Autodesk Inventor part; units mm, degrees
ref_plane "YZ Plane" through (0, 0, 0) normal (1, 0, 0) x (0, 1, 0)
ref_plane "XZ Plane" through (0, 0, 0) normal (0, 1, 0) x (-1, 0, 0)
ref_plane "XY Plane" through (0, 0, 0) normal (0, 0, 1) x (1, 0, 0)
sketch "スケッチ1" plane through (0, 0, 0) normal (0, 0, 1) x (1, 0, 0)
  line L0 (-341.5, 417.85) -> (341.5, 417.85)
  line L1 (341.5, 417.85) -> (341.5, -417.85)
  line L2 (341.5, -417.85) -> (-341.5, -417.85)
  line L3 (-341.5, -417.85) -> (-341.5, 417.85)
  line L4 (-478.1, 0) -> (478.1, 0)
  line L5 (0, -584.99) -> (0, 584.99)
  point P0 (0, 0)
  point P1 (341.5, 0)
  point P2 (0, 417.85)
  dimension "d2" = 835.7
  dimension "d3" = 683
extrude "押し出し1" add sketch "スケッチ1" along normal blind 1357
sketch "スケッチ3" plane through (0, 0, 0) normal (0, 0, 1) x (1, 0, 0)
  line L0 (-171.5, 417.85) -> (171.5, 417.85)
  line L1 (171.5, 417.85) -> (341.5, -132.15)
  line L2 (341.5, -132.15) -> (341.5, -166.8)
  line L3 (341.5, -166.8) -> (135, -417.85)
  line L4 (-341.5, 417.85) -> (341.5, 417.85)
  line L5 (341.5, 417.85) -> (341.5, -417.85)
  line L6 (341.5, -417.85) -> (-341.5, -417.85)
  line L7 (0, -595.6665) -> (0, 649.0488)
  line L8 (135, -417.85) -> (0, -417.85)
  line L9 (-341.5, -417.85) -> (341.5, -417.85)
  line L10 (-171.5, 417.85) -> (-341.5, -132.15)
  line L11 (-341.5, -132.15) -> (-341.5, -166.8)
  line L12 (-341.5, -166.8) -> (-135, -417.85)
  line L13 (-135, -417.85) -> (0, -417.85)
  line L14 (341.5, 417.85) -> (-341.5, 417.85)
  line L15 (171.5, 417.85) -> (341.5, 417.85)
  line L16 (341.5, 417.85) -> (341.5, -132.15)
  line L17 (341.5, -417.85) -> (341.5, 417.85)
  line L18 (341.5, -166.8) -> (341.5, -417.85)
  line L19 (341.5, -417.85) -> (135, -417.85)
  line L20 (-135, -417.85) -> (-341.5, -417.85)
  line L21 (-341.5, -417.85) -> (-341.5, -166.8)
  line L22 (-341.5, 417.85) -> (-341.5, -417.85)
  line L23 (-171.5, 417.85) -> (-341.5, 417.85)
  line L24 (-341.5, -132.15) -> (-341.5, 417.85)
  point P0 (0, 0)
  point P1 (0, 417.85)
  dimension "d9" = 343
  dimension "d10" = 34.65
  dimension "d11" = 550
  dimension "d12" = 206.5
extrude "押し出し2" cut sketch "スケッチ3" along normal through all both and the other way through all contours L10 L22 L4 | L4 L5 L1 | L12 L6 L21 | L3 L5 L6
sketch "スケッチ5" plane through (0, 0, 1357) normal (0, 0, 1) x (1, 0, 0)
  line L0 (-171.5, 417.85) -> (-341.5, -132.15)
  line L1 (-341.5, -132.15) -> (-171.5, 417.85)
  line L2 (171.5, 417.85) -> (-171.5, 417.85)
  line L3 (-171.5, 417.85) -> (171.5, 417.85)
  line L4 (341.5, -132.15) -> (171.5, 417.85)
  line L5 (171.5, 417.85) -> (341.5, -132.15)
  line L6 (341.5, -132.15) -> (-341.5, -132.15)
  point P0 (0, 0)
extrude "押し出し3" cut sketch "スケッチ5" against normal blind 1337
sketch "スケッチ6" plane through (-341.5, -132.15, 1357) normal (0, 1, 0) x (1, 0, 0)
  line L0 (0, 1265.7) -> (0, 665.7)
  line L1 (0, 665.7) -> (76.7, 665.7)
  line L2 (76.7, 665.7) -> (0, 1265.7)
  line L3 (0, 1357) -> (170, 1357)
  line L4 (0, 0) -> (0, 1337)
  line L5 (341.5, 1357) -> (341.5, 1610.7019)
  line L6 (683, 1265.7) -> (683, 665.7)
  line L7 (683, 665.7) -> (606.3, 665.7)
  line L8 (606.3, 665.7) -> (683, 1265.7)
  line L9 (0, 665.7) -> (76.7, 665.7)
  line L10 (0, 665.7) -> (0, 0)
  line L11 (0, 1357) -> (0, 0)
  line L12 (76.7, 665.7) -> (122.641, 0)
  line L13 (206.5, 0) -> (206.5, 1357)
  line L14 (0, 0) -> (122.641, 0)
  line L15 (683, 0) -> (0, 0)
  line L16 (683, 665.7) -> (606.3, 665.7)
  line L17 (683, 665.7) -> (606.3, 665.7)
  line L18 (683, 665.7) -> (683, 0)
  line L19 (606.3, 665.7) -> (560.359, 0)
  line L20 (683, 0) -> (560.359, 0)
  point P0 (683, 0)
  dimension "d17" = 91.3
  dimension "d18" = 600
  dimension "d19" = 76.7
  dimension "d21" = 45.941
extrude "押し出し4" cut sketch "スケッチ6" against normal through all
sketch "スケッチ7" plane through (0, 0, 0) normal (1, 0, 0) x (0, 1, 0)
  line L0 (-315.8994, 1357) -> (-417.85, 1357)
  line L1 (-371.05, 1357) -> (-417.85, 1357)
  line L2 (-417.85, 1357) -> (-417.85, 799.8485)
  line L3 (-417.85, 1357) -> (-417.85, 0)
  line L4 (-417.85, 799.8485) -> (-371.05, 862.4972)
  line L5 (-371.05, 862.4972) -> (-371.05, 1357)
  line L6 (-315.8994, 1357) -> (-260.0471, 691.3)
  line L7 (-417.85, 0) -> (-417.85, 1357)
  point P0 (0, 0)
  dimension "d25" = 143.239
  dimension "d26" = 46.8
extrude "押し出し5" cut sketch "スケッチ7" along normal through all both and the other way through all
sketch "スケッチ8" plane through (0, 0, 0) normal (1, 0, 0) x (0, 1, 0)
  line L0 (-132.15, 20) -> (417.85, 20)
  line L1 (167.85, 20) -> (-132.15, 252.8315)
  line L2 (-132.15, 91.3) -> (-132.15, 691.3)
  line L3 (-132.15, 20) -> (-132.15, 91.3)
  line L4 (-132.15, 252.8315) -> (-132.15, 20)
  line L5 (-132.15, 20) -> (167.85, 20)
  point P0 (0, 0)
  dimension "d29" = 37.815
  dimension "d30" = 300
extrude "押し出し6" add sketch "スケッチ8" along normal mid plane 400
sketch "スケッチ9" plane through (0, 0, 0) normal (1, 0, 0) x (0, 1, 0)
  line L0 (159.383, 0) -> (-34.9495, -326.55)
  line L1 (-34.9495, -326.55) -> (-365.0355, -370.5068)
  line L2 (-365.0355, -370.5068) -> (-417.85, 0)
  line L3 (-772.2018, 0) -> (616.192, 0)
  line L4 (-417.85, 0) -> (-417.85, 799.8485)
  point P0 (0, 0)
  dimension "d33" = 171.887
  dimension "d34" = 128.343
  dimension "d35" = 90.527
  dimension "d36" = 380
  dimension "d37" = 333
extrude "押し出し7" add sketch "スケッチ9" along normal mid plane 400
sketch "スケッチ10" plane through (0, 0, 0) normal (0, 0, 1) x (1, 0, 0)
  line L0 (-200, -338.827) -> (-341.5, -166.8)
  line L1 (-200, -365.0355) -> (-200, -417.85)
  line L2 (-200, -338.827) -> (-200, -417.85)
  line L3 (-135, -417.85) -> (-200, -417.85)
  line L4 (-200, -417.85) -> (-135, -417.85)
  line L5 (-135, -417.85) -> (-200, -338.827)
  line L6 (200, -338.827) -> (200, 159.383)
  line L7 (200, -338.827) -> (135, -417.85)
  line L8 (200, -338.827) -> (135, -417.85)
  line L9 (200, -417.85) -> (135, -417.85)
  line L10 (135, -417.85) -> (200, -417.85)
  line L11 (200, -417.85) -> (200, -338.827)
  point P0 (0, 0)
extrude "押し出し8" cut sketch "スケッチ10" against normal through all
properties part number "newbody"
Verification items for the finished model (mm, model axes). A direction names the side the tool comes from. Give positions to 0.01 mm unless a question says otherwise; leave off trailing zeros. Loops run counter-clockwise (first coordinate to the right, second up) from the corner with the lowest first, then second, coordinate; pieces in that order, holes last.
1) Set-up check for faces 1 (the flat face through (200, -149, -140)), 2 (the flat face through (-5, 213, 0)), 3 (the flat face through (200, -51, 86)), 4 (the flat face through (-5, 208, 20)): record each of +Z, -Z, +X, -X, +Y, -Y from which the full face is reachable in a straight line by a thin tool's end or side.
2) Thickness scan on line 1 along Z through (x, y) = (269, -98.5); line 2 along Y through (x, z) = (24.5, 653.5); line 3 along Y through (x, z) = (-154.5, 1282). Record the ranges inside material, lowest first.
3) Sectioned sample at A-A, the plane y = -16.5. Enter the section's corners in (x, z).
4) Depth check by flat-ended pin: pin 1 Ø10 at (y, z) = (-260.5, 18.5) entering from +X; pin 2 Ø12 at (x, z) = (-166.5, 1056) entering from -Y; pin 3 Ø5 at (x, y) = (-70, -12) entering from +Z. Enter the tip coordinate at first touch or a pass-through.
5) Sectioned sample at D-D, the plane z = 625. Enter the section's corners in (x, y).
6) Sectioned sample at B-B, the plane x = 74. Enter the section's corners in (y, z), then the cut area to 3 significant figures.
7) Sectioned sample at C-C, the plane z = 204. Enter the section's corners in (x, y), then the cut area to 3 significant figures.
Answers:
1. face 1: -Z, +X, +Y, -Y
1. face 2: -Z, +Y
1. face 3: +Z, +X, +Y
1. face 4: +Z, +Y
2. line 1: z = 0 to 20
2. line 2: y = -417.85 to -132.15
2. line 3: y = -371.05 to -132.15
3. outline: (-305.75, 0) - (-200, 0) - (-200, -295.55) - (200, -295.55) - (200, 0) - (305.75, 0) - (305.75, 20) - (200, 20) - (200, 163.07) - (-200, 163.07) - (-200, 20) - (-305.75, 20) - close
4. pin 1: stops at x = 268.54
4. pin 2: stops at y = -371.05
4. pin 3: stops at z = 161.52
5. outline: (-273.28, -249.74) - (-135, -417.85) - (135, -417.85) - (273.28, -249.74) - (273.28, -132.15) - (-273.28, -132.15) - close
6. outline: (-417.85, 0) - (-365.04, -370.51) - (-34.95, -326.55) - (159.38, 0) - (417.85, 0) - (417.85, 20) - (167.85, 20) - (-132.15, 252.83) - (-132.15, 1357) - (-371.05, 1357) - (-371.05, 862.5) - (-417.85, 799.85) - close
6. area: 566,000 mm2
7. outline: (-327.09, -184.31) - (-135, -417.85) - (135, -417.85) - (327.09, -184.31) - (327.09, -132.15) - (200, -132.15) - (200, -69.23) - (-200, -69.23) - (-200, -132.15) - (-327.09, -132.15) - close
7. area: 167,000 mm2
